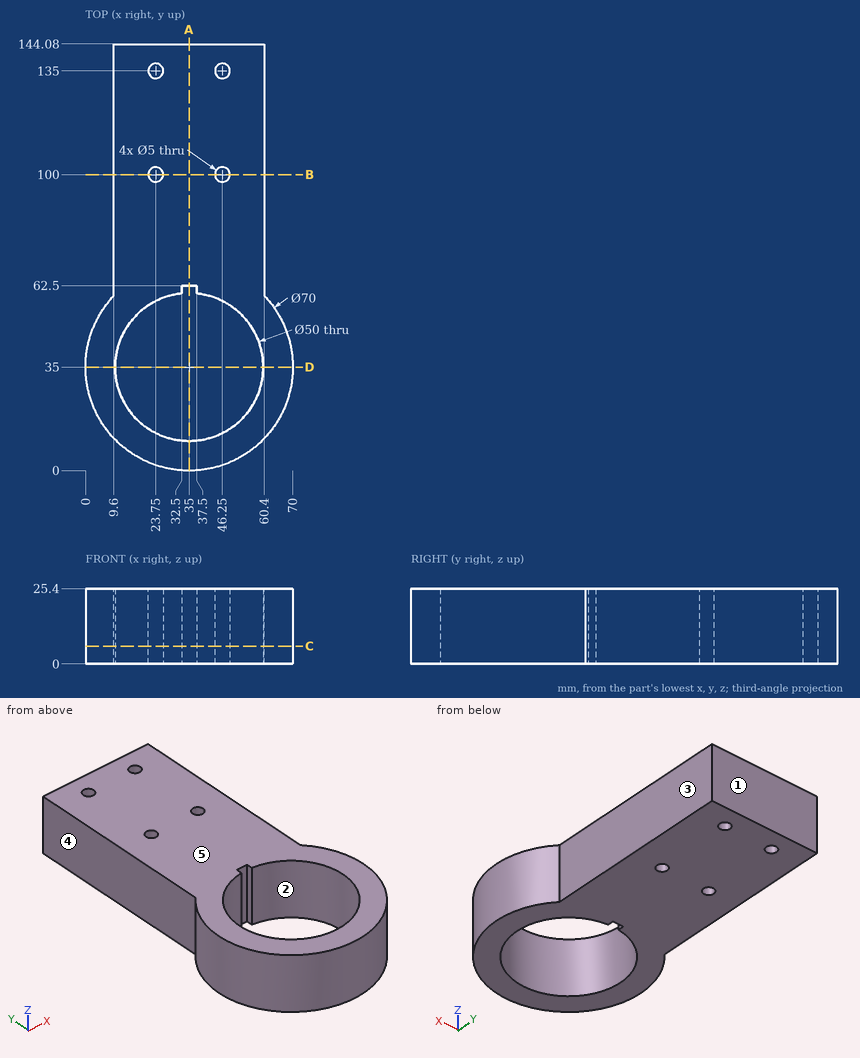
The drawing under review shows one solid part. Ordinate dimensions are in mm from its lowest x, y, z. A direction names the side the tool comes from. Give positions to 0.01 mm unless a question says otherwise; leave off trailing zeros. Order: outer loops, then holes, each group sorted by start corner. A loop starts at its lowest first (then second) coordinate and runs counter-clockwise, first axis right, second up. Notation, with made-up numbers: (44.5, -9) -> (75.5, -9) arc R11 cw to (75.5, -3) -> close; hole circle Ø6 at (89, -14). An arc over 180 degrees is marked (long way). Write item = value, one per line.
1) Draft analysis for pull direction Y (two halves, no side actions). For the marked faces 1, 2 and 3, state which applies: pulls with the +Y half, pulls with the -Y half, needs draft (parallel to the pull), parting line crosses it, or undercut.
Findings:
face_1 = pulls with the +Y half
face_2 = undercut
face_3 = needs draft
2) For the marked faces 4 and 5, list the 3-axis set-ups (+Z, -Z, +X, -X, +Y, -Y) from which the entire face can be reached by the end or side of a thin tool; tool diameter is ignored.
Findings:
face_4 = +Z, -Z, -X, +Y
face_5 = +Z, +X, -X, +Y, -Y
3) Insertion check: pin 1 (2 mm diameter, centred on x = 33.5, y = 122.5, fed in from -Z); pin 2 (12.5 mm diameter, centred on y = 107.5, z = 19, fed in from +X); pin 3 (1 mm diameter, centred on y = 113.5, z = 10.5, fed in from -X); pin 4 (4 mm diameter, centred on x = 53.5, z = 6, fed in from -Y). Each pin has a flat end and moves straight along its axis. Give the tip position at first contact, or say it passes through.
Findings:
pin_1 = 0
pin_2 = 60.4
pin_3 = 9.6
pin_4 = 4.13
4) We need section A-A, the plane x = 35. Give the boundary of the cut face in (y, z).
Findings:
outline = (0, 0) -> (10, 0) -> (10, 25.4) -> (0, 25.4) -> close; (62.5, 0) -> (144.08, 0) -> (144.08, 25.4) -> (62.5, 25.4) -> close
5) To check wall thickness, follow L1, parallel to X at y = 135, z = 16; L2, parallel to Y at x = 35, z = 7; L3, parallel to Y at x = 46.25, z = 15. State the ranges of each line that lie inside material, in increasing order. Write a range as from..to.
Findings:
L1 = 9.6..21.25, 26.25..43.75, 48.75..60.4
L2 = 0..10, 62.5..144.08
L3 = 1.86..12.67, 57.33..97.5, 102.5..132.5, 137.5..144.08
6) We need section C-C, the plane z = 6. Give the boundary of the cut face in (x, y), and give its area (3 significant figures).
Findings:
outline = (9.6, 59.08) arc R35 ccw (long way) to (60.4, 59.08) -> (60.4, 144.08) -> (9.6, 144.08) -> close; hole circle Ø5 at (23.75, 100); hole circle Ø5 at (23.75, 135); hole (32.5, 59.87) arc R25 ccw (long way) to (37.5, 59.87) -> (37.5, 62.5) -> (32.5, 62.5) -> close; hole circle Ø5 at (46.25, 100); hole circle Ø5 at (46.25, 135)
area = 5,730 mm^2
7) We need section B-B, the plane y = 100. Give the boundary of the cut face in (x, z), and give its area (3 significant figures).
Findings:
outline = (9.6, 0) -> (21.25, 0) -> (21.25, 25.4) -> (9.6, 25.4) -> close; (26.25, 0) -> (43.75, 0) -> (43.75, 25.4) -> (26.25, 25.4) -> close; (48.75, 0) -> (60.4, 0) -> (60.4, 25.4) -> (48.75, 25.4) -> close
area = 1,040 mm^2
8) We need section D-D, the plane y = 35. Give the boundary of the cut face in (x, z).
Findings:
outline = (0, 0) -> (10, 0) -> (10, 25.4) -> (0, 25.4) -> close; (60, 0) -> (70, 0) -> (70, 25.4) -> (60, 25.4) -> close
